Check sheet for the drawn part. Datum: minimum x, y, z corner. Units: mm. A direction names the side the tool comes from. Coordinates: 2 decimals unless noted, no trailing zeros. Write each loop counter-clockwise with the first axis right and the second up, starting at its lowest first coordinate (ties: lowest second). Pieces come first, ordered by that corner, then holes. Notation, with made-up numbers: (89.25, 23.5) -> (138.25, 23.5) arc R18 ccw to (138.25, 52.5) -> close; hole circle Ø10 at (64, 1). An arc over 180 degrees is marked (long way). Answer in a Markdown table with one row per item. Add a question column.
1. Cross-section at A-A on y = 6. Record the cut outline in (x, z), and give its area (3 significant figures).
2. Cross-section at D-D on x = 15.5. Record the cut outline in (y, z), and give its area (3 significant figures).
3. Depth check by flat-ended pin: P1, Ø1.5, axis at x = 14.5, z = 7.5, coming from the +Y side; P2, Ø4, axis at x = 15.5, y = 5.5, coming from the -Z side; P3, Ø4, axis at x = 9.5, z = 8.5, coming from the +Y side. Enter the tip coordinate at first touch or a pass-through.
4. Set-up check for the marked faces 1, 2 and 3: record each of +Z, -Z, +X, -X, +Y, -Y from which the full face is reachable in a straight line by a thin tool's end or side.
5. Scan lines: L1, parallel to Z at x = 1.5, y = 4; L2, parallel to X at y = 8.75, z = 2.25; L3, parallel to Y at x = 5.5, z = 6.25. Record each from-to range of solid material in increasing order. Write a range as from..to.
6. Cross-section at C-C on x = 7.5. Record the cut outline in (y, z).
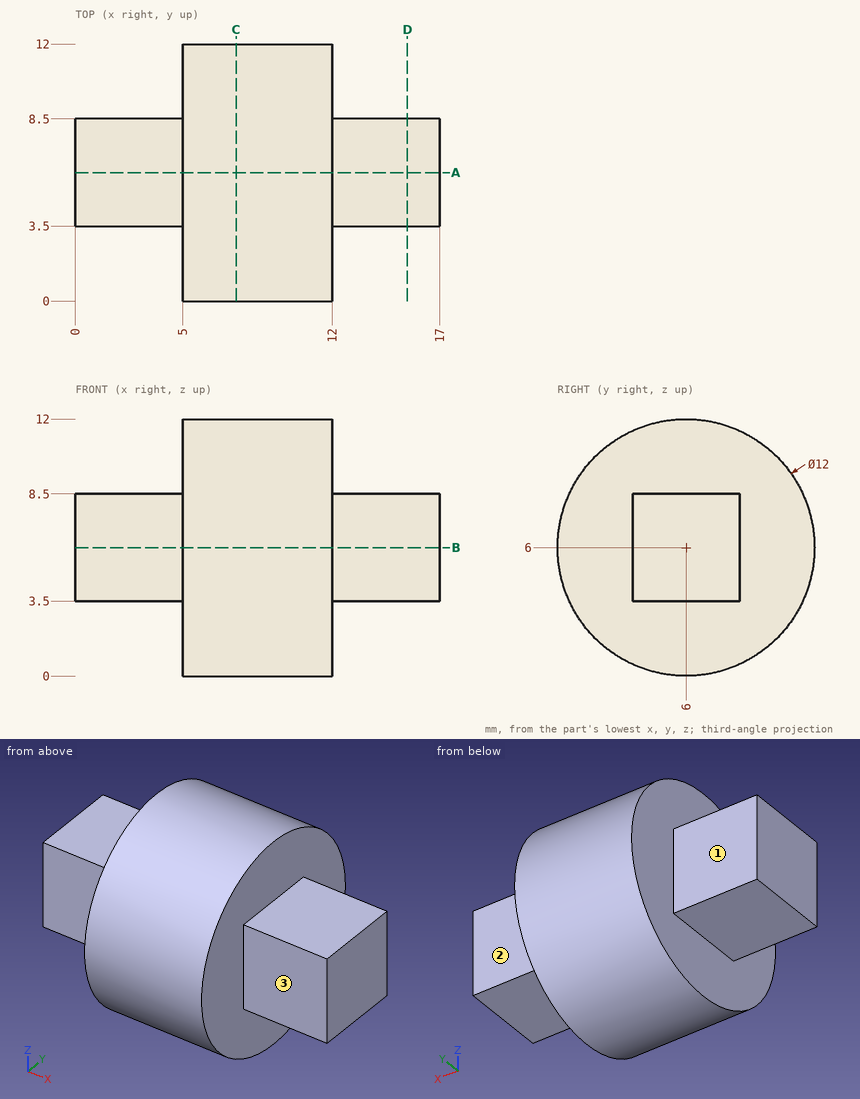
Results found:
| question | item | result |
|---|---|---|
| 1 | outline | (0, 3.5) -> (5, 3.5) -> (5, 0) -> (12, 0) -> (12, 3.5) -> (17, 3.5) -> (17, 8.5) -> (12, 8.5) -> (12, 12) -> (5, 12) -> (5, 8.5) -> (0, 8.5) -> close |
| 1 | area | 134 mm^2 |
| 2 | outline | (3.5, 3.5) -> (8.5, 3.5) -> (8.5, 8.5) -> (3.5, 8.5) -> close |
| 2 | area | 25.0 mm^2 |
| 3 | P1 | stops at y = 8.5 |
| 3 | P2 | stops at z = 3.5 |
| 3 | P3 | stops at y = 11.98 |
| 4 | face 1 | +Z, -Z, -X, +Y |
| 4 | face 2 | +Z, -Z, +X, +Y |
| 4 | face 3 | +Z, -Z, +X, -Y |
| 5 | L1 | z = 3.5..8.5 |
| 5 | L2 | x = 5..12 |
| 5 | L3 | y = 0.01..11.99 |
| 6 | outline | circle Ø12 at (6, 6) |
